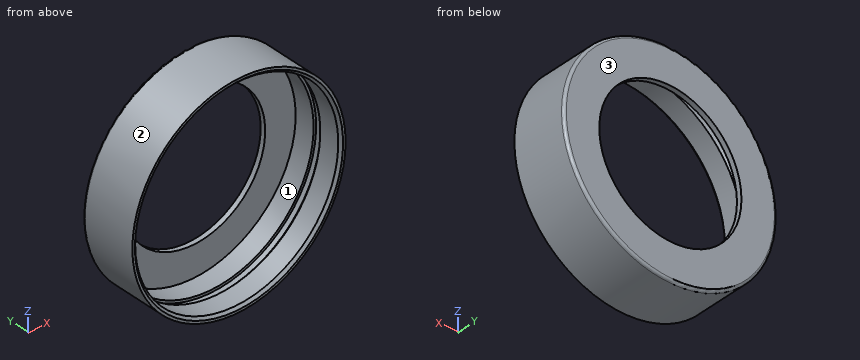
from build123d import *

# Parameters (mm, degrees)
FILETE1_R = 0.5


with BuildPart() as part:
    # Esboço1 → Revolução2 (revolve)
    with BuildSketch(Plane.XY):
        Polygon((-21, 0), (-21, 11), (-14, 11), (-14, 10), (-20, 10), (-20, 6), (-20.5, 6), (-20.5, 5), (-20, 4.5), (-20, 0.5), (-20.5, 0), align=None)
    revolve(axis=Axis((0, 0, 0), (0, 1, 0)))

    # Filete1
    filete1_edges = [part.edges().sort_by_distance(p)[0] for p in [
        (21, 11, 0),
    ]]
    fillet(filete1_edges, radius=FILETE1_R)


solid = part.part
Build history of the part. All positions in model axes, mm. Face numbers are marked on the shaded views. Give positions to 0.01 mm unless a question says otherwise; leave off trailing zeros. Loops run counter-clockwise (first coordinate to the right, second up) from the corner with the lowest first, then second, coordinate; pieces in that order, holes last. Notation, with made-up numbers: (28, 12.5) - (32, 12.5) arc R13 cw to (32, 20.5) - close; hole circle Ø8 at (-8.75, -16). An arc over 180 degrees is marked (long way). Write item = value, one per line. Start each with the question number.
1) Pull direction Z, two halves, no side cores. Call the marked faces 1, 2 and 3: +Z half, -Z half, draft (parallel to the pull), parting line (faces both ways), or undercut.
2) Band-saw the part on A-A on x = 0. Give the cut face in (y, z).
3) Band-saw the part on C-C on y = 2.75. Give the cut face in (x, z).
4) Band-saw the part on B-B on z = 0. Give the cut face in (x, y), plus the area to 3 significant figures.
5) Drop flat-ended pins along their axis: pin 1 Ø2 at (x, y) = (-1.5, 2) entering from -Z; pin 2 Ø2 at (x, y) = (-7.5, 3.5) entering from +Z; pin 3 Ø1 at (y, z) = (2, 14) entering from -X. Give the stop position or say it passes through.
6) Probe probe 1 along Z at (x, y) = (0, 5.6); probe 2 along Z at (x, y) = (0, 10.55); probe 3 along X at (y, z) = (10.25, 0.5). List the from-to ranges inside material, lowest first. Write a range as from..to.
Final values:
q1.face_1 = undercut
q1.face_2 = parting line
q1.face_3 = draft
q2.outline = (0, -21) - (10.5, -21) arc R0.5 ccw to (11, -20.5) - (11, -14) - (10, -14) - (10, -20) - (6, -20) - (6, -20.5) - (5, -20.5) - (4.5, -20) - (0.5, -20) - (0, -20.5) - close; (0, 20.5) - (0.5, 20) - (4.5, 20) - (5, 20.5) - (6, 20.5) - (6, 20) - (10, 20) - (10, 14) - (11, 14) - (11, 20.5) arc R0.5 ccw to (10.5, 21) - (0, 21) - close
q3.outline = circle Ø42 at (0, 0); hole circle Ø40 at (0, 0)
q4.outline = (-21, 0) - (-20.5, 0) - (-20, 0.5) - (-20, 4.5) - (-20.5, 5) - (-20.5, 6) - (-20, 6) - (-20, 10) - (-14, 10) - (-14, 11) - (-20.5, 11) arc R0.5 ccw to (-21, 10.5) - close; (14, 10) - (20, 10) - (20, 6) - (20.5, 6) - (20.5, 5) - (20, 4.5) - (20, 0.5) - (20.5, 0) - (21, 0) - (21, 10.5) arc R0.5 ccw to (20.5, 11) - (14, 11) - close
q4.area = 32.4 mm²
q5.pin_1 = -20.99
q5.pin_2 = 19.97
q5.pin_3 = -16.09
q6.probe_1 = -21..-20.5, 20.5..21
q6.probe_2 = -21..-14, 14..21
q6.probe_3 = -20.99..-13.99, 13.99..20.99
